Design review of the part built by this model. Coordinates are the model's own, in mm. Face numbers are marked on the shaded views. A direction names the side the tool comes from. Round coordinates to 2 decimals unless told otherwise and drop trailing zeros. Loops run counter-clockwise (first coordinate to the right, second up) from the corner with the lowest first, then second, coordinate; pieces in that order, holes last. Notation, with made-up numbers: (-23, 85) - (-18, 85) arc R26 ccw to (-18, 106) - close; hole circle Ø4 at (30.5, 69). An arc over 180 degrees is marked (long way). Return JSON: item names as keys, results as strings. Group by question number.
(1) We need section A-A, the plane z = 78.75. Write out the cut boundary in (x, y), and give its area (3 significant figures).
(2) We need section D-D, the plane z = 56. Write out the cut boundary in (x, y).
(3) Clearance check with flat-ended pins moving along their axes: pin 1 (5 mm diameter, centred on x = 6.5, y = 28, fed in from +Z); pin 2 (16.5 mm diameter, centred on y = 27, z = 17.5, fed in from +X); pin 3 (1.5 mm diameter, centred on x = 2.5, z = -51.5, fed in from +Y). State where each tip first meets the part, or that it passes through.
(4) We need section C-C, the plane z = 13. Write out the cut boundary in (x, y), and give its area (3 significant figures).
(5) For the marked faces 1 and 2, list the 3-axis set-ups (+Z, -Z, +X, -X, +Y, -Y) from which the entire face can be reached by the end or side of a thin tool; tool diameter is ignored.
(6) We need section B-B, the plane y = 30. Write out the cut boundary in (x, z).
(7) Wall thickness on L1, parallel to Z at x = 0.6, y = 30; L2, parallel to Z at x = 4.75, y = 26; L3, parallel to Y at x = 0.2, z = 35: over which ranges is each line inside the solid? List them lowest first. Write a range as [from, to].
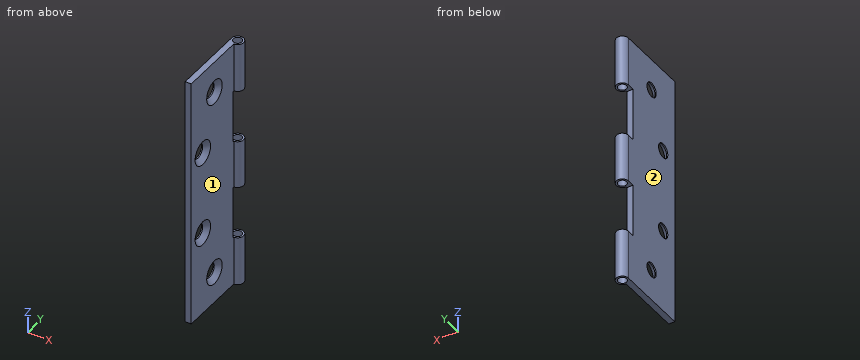
from build123d import *

# Parameters (mm, degrees)
SKETCH_1_W                  = 5
SKETCH_1_H                  = 60
EXTRUDE_2_DEPTH             = 105
SKETCH_2_R                  = 5
SKETCH_3_R                  = 3.5
CUT_EXTRUDE_1_DEPTH         = 221.056810847
HOLE_WIZARD_M101_AT_2_COUNT = 2
HOLE_WIZARD_M101_AT_2_PITCH = 46.25
VIR_2_DEPTH                 = 124.592070943
VIR_2_DEPTH_BACK            = 124.592070943
SKETCH_12_W                 = 44
SKETCH_12_H                 = 11


with BuildPart() as part:
    # Эскиз1 → Вытянуть-Тонкостенный2 (new, symmetric)
    with BuildSketch(Plane.XY):
        with Locations((2.5, 30)):
            Rectangle(SKETCH_1_W, SKETCH_1_H)
    extrude(amount=EXTRUDE_2_DEPTH, both=True)

    # По траектории1: sweep along a curve in space
    with BuildLine() as sweep_1_path:
        Line((0, 60, 105), (0, 60, -105))
    # Эскиз2 → По траектории1 (sweep)
    with BuildSketch(Plane.XY.offset(105)):
        with Locations((5, 60)):
            Circle(SKETCH_2_R)
    sweep(path=sweep_1_path.line)

    # Эскиз3 → Вырез-Вытянуть1 (cut, through all)
    with BuildSketch(Plane.XY.offset(105)):
        with Locations((5, 60)):
            Circle(SKETCH_3_R)
    extrude(amount=-CUT_EXTRUDE_1_DEPTH, mode=Mode.SUBTRACT)

    # Эскиз8 → Зенковка для  винта с плоской головкой M101 (revolve, cut)
    with BuildSketch(Plane(origin=(5, 30, 78.75), x_dir=(0, 0, -1), z_dir=(0, 1, 0))):
        Polygon((0, 0), (0, 5), (6, 5), (6, 4), (10, 0), align=None)
    hole_wizard_m101 = revolve(axis=Axis((11.35, 30, 78.75), (-1, 0, 0)), mode=Mode.SUBTRACT)

    # Зенковка для  винта с плоской головкой M101 at 2: Зенковка для  винта с плоской головкой M101 ×2
    with Locations(*[Vector(0, -0.3243243243243243, -0.945945945945946) * (i * HOLE_WIZARD_M101_AT_2_PITCH) for i in range(1, HOLE_WIZARD_M101_AT_2_COUNT)]):
        add(hole_wizard_m101, mode=Mode.SUBTRACT)

    # Зеркальное отражение1: Зенковка для  винта с плоской головкой M101 across plane
    add(hole_wizard_m101.mirror(Plane.XY), mode=Mode.SUBTRACT)

    # Зеркальное отражение1 copy 1 sketch → Зеркальное отражение1 copy 1 (revolve, cut)
    with BuildSketch(Plane(origin=(5, 15, -35), x_dir=(0, 0, 1), z_dir=(0, 1, 0))):
        Polygon((0, 0), (0, -5), (6, -5), (6, -4), (10, 0), align=None)
    revolve(axis=Axis((11.35, 15, -35), (1, 0, 0)), mode=Mode.SUBTRACT)

    # Эскиз12 → vir_2 (cut, two sides: drawn at the far end of the back side and taken through both)
    with BuildSketch(Plane(origin=(5, 0, 0), x_dir=(0, 0, -1), z_dir=(1, 0, 0)).offset(-VIR_2_DEPTH_BACK)):
        with Locations((-42, 59.5)):
            Rectangle(SKETCH_12_W, SKETCH_12_H)
        with Locations((42, 59.5)):
            Rectangle(SKETCH_12_W, SKETCH_12_H)
    extrude(amount=VIR_2_DEPTH + VIR_2_DEPTH_BACK, mode=Mode.SUBTRACT)


solid = part.part
Solutions:
{
 "1": {"outline": "(0, 0) - (5, 0) - (5, 20) - (1, 24) - (0, 24) - close; (0, 36) - (1, 36) - (5, 40) - (5, 55) arc R5 ccw (long way) to (0, 60) - close; hole circle Ø7 at (5, 60)", "area": "244 mm^2"},
 "2": {"outline": "(0, 0) - (5, 0) - (5, 54) - (0, 54) - close"},
 "3": {"pin 1": "z = 105", "pin 2": "x = 5", "pin 3": "y = 54"},
 "4": {"outline": "(0, 0) - (5, 0) - (5, 55) arc R5 ccw (long way) to (0, 60) - close; hole circle Ø7 at (5, 60)", "area": "320 mm^2"},
 "5": {"face 1": "+Z, -Z, +X, -Y", "face 2": "+Z, -Z, -X, +Y, -Y"},
 "6": {"outline": "(0, -105) - (5, -105) - (5, -88.75) - (1, -84.75) - (0, -84.75) - close; (0, -72.75) - (1, -72.75) - (5, -68.75) - (5, 68.75) - (1, 72.75) - (0, 72.75) - close; (0, 84.75) - (1, 84.75) - (5, 88.75) - (5, 105) - (0, 105) - close"},
 "7": {"L1": "[-105, -84.75], [-72.75, 72.75], [84.75, 105]", "L2": "[-105, -87.64], [-69.86, 69.86], [87.64, 105]", "L3": "[0, 9], [21, 54]"}
}
